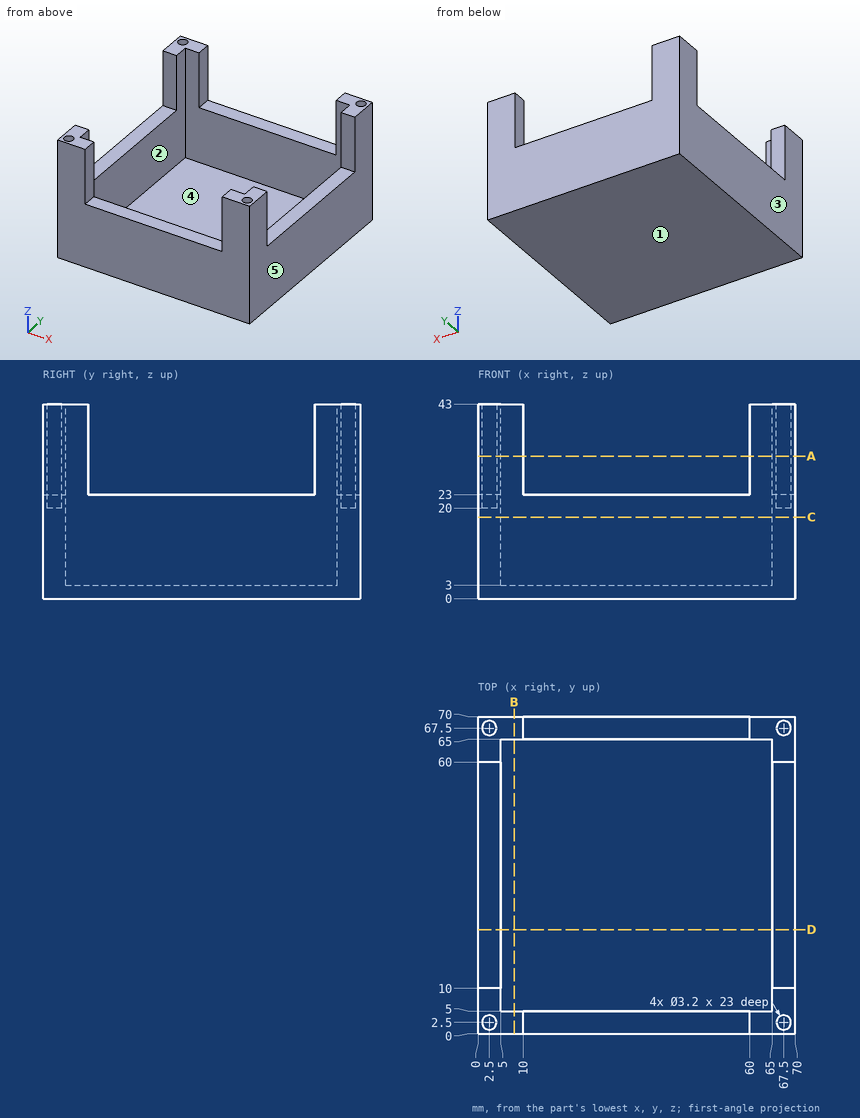
Input: dimensioned drawing with shaded views. Units: mm. Origin: part minimum x, y, z. A direction names the side the tool comes from. Give positions to 0.01 mm unless a question says otherwise; leave off trailing zeros. Loops run counter-clockwise (first coordinate to the right, second up) from the corner with the lowest first, then second, coordinate; pieces in that order, holes last. Notation, with made-up numbers: M 68,-5.5 L 100,-5.5 A30 cw 100,21.5 Z; hole C -6,35 d3. An arc over 180 degrees is marked long. Put each result on its own line as item: value.
1) First-contact query: P1, Ø1.6, axis at x = 3, y = 2.5, coming from the +Z side; P2, Ø10, axis at x = 43.5, y = 21, coming from the -Z side; P3, Ø1.5, axis at x = 36, y = 2.5, coming from the +Z side. Flat tips, straight axial feed; report the tip coordinate or a pass-through.
Computed values:
P1: stops at z = 20
P2: stops at z = 0
P3: stops at z = 23
2) Material intervals for L1, parallel to X at y = 67.5, z = 32.75; L2, parallel to Y at x = 63, z = 27; L3, parallel to X at y = 67, z = 32, sorted ascending. Write a range as from..to.
Computed values:
L1: x = 0..0.9, 4.1..10, 60..65.9, 69.1..70
L2: y = 0..5, 65..70
L3: x = 0..0.98, 4.02..10, 60..65.98, 69.02..70
3) Cut plane B-B, the plane x = 8. Return the cut outline in (y, z), plus the area to 3 significant figures.
Computed values:
outline: M 0,0 L 70,0 L 70,43 L 65,43 L 65,3 L 5,3 L 5,43 L 0,43 Z
area: 610 mm^2
4) Cut plane D-D, the plane y = 23. Return the cut outline in (x, z).
Computed values:
outline: M 0,0 L 70,0 L 70,23 L 65,23 L 65,3 L 5,3 L 5,23 L 0,23 Z
5) Cut plane A-A, the plane z = 31.5. Return the cut outline in (x, y), plus the area to 3 significant figures.
Computed values:
outline: M 0,0 L 10,0 L 10,5 L 5,5 L 5,10 L 0,10 Z; M 0,60 L 5,60 L 5,65 L 10,65 L 10,70 L 0,70 Z; M 60,0 L 70,0 L 70,10 L 65,10 L 65,5 L 60,5 Z; M 60,65 L 65,65 L 65,60 L 70,60 L 70,70 L 60,70 Z; hole C 2.5,2.5 d3.2; hole C 2.5,67.5 d3.2; hole C 67.5,2.5 d3.2; hole C 67.5,67.5 d3.2
area: 268 mm^2
6) Cut plane C-C, the plane z = 18. Return the cut outline in (x, y), plus the area to 3 significant figures.
Computed values:
outline: M 0,0 L 70,0 L 70,70 L 0,70 Z; hole M 5,5 L 65,5 L 65,65 L 5,65 Z
area: 1,300 mm^2
7) Mould query, pull axis X, two halves, no side actions, for the marked faces 3, 4 and 5. Classes: released by +X, released by -X, zero draft, split by the parting line, or undercut.
Computed values:
face 3: released by -X
face 4: undercut
face 5: released by +X
8) Reachability of the marked faces 1 and 2 from +Z, -Z, +X, -X, +Y, -Y: full face, straight path, thin tool, end or side. Return the list, or none.
Computed values:
face 1: -Z, +X, -X, +Y, -Y
face 2: +Z
